from build123d import *

# Parameters (mm, degrees)
EXTRUDE_1_DEPTH = 2


with BuildPart() as part:
    # 草图1 → 凸台-拉伸1 (new body)
    with BuildSketch(Plane.XY):
        with BuildLine():
            Line((-8.45, -5.2), (-8.45, -7))
            Line((-8.45, -7), (12.741644056, -7))
            Line((12.741644056, -7), (13.101478198, -6.889754544))
            Line((13.101478198, -6.889754544), (14.486104816, -6.144709151))
            Line((14.486104816, -6.144709151), (15.312149212, -5.46294768))
            Line((15.312149212, -5.46294768), (14.987866566, -4.436878246))
            Line((14.987866566, -4.436878246), (16.015719748, -4.755461916))
            ThreePointArc((16.015719748, -4.755461916), (17.441105489, -2.542698595), (17.984281104, 0.032763748))
            Line((17.984281104, 0.032763748), (17.029669504, 0.531416269))
            Line((17.029669504, 0.531416269), (17.981499226, 1.035358552))
            ThreePointArc((17.981499226, 1.035358552), (17.266800727, 3.051396039), (15.995852657, 4.771829734))
            Line((15.995852657, 4.771829734), (14.969602225, 4.448120344))
            Line((14.969602225, 4.448120344), (15.288760048, 5.475795391))
            Line((15.288760048, 5.475795391), (14.459323359, 6.1534255))
            Line((14.459323359, 6.1534255), (13.070995905, 6.891551848))
            Line((13.070995905, 6.891551848), (12.710615967, 7))
            Line((12.710615967, 7), (-8.45, 7))
            Line((-8.45, 7), (-8.45, 5.2))
            ThreePointArc((-8.45, 5.2), (-8.308578644, 4.858578644), (-8.65, 5))
            Line((-8.65, 5), (-10.35, 5))
            ThreePointArc((-10.35, 5), (-10.691421356, 4.858578644), (-10.55, 5.2))
            Line((-10.55, 5.2), (-10.55, 7))
            Line((-10.55, 7), (-13, 7))
            Line((-13, 7), (-13, -7))
            Line((-13, -7), (-10.55, -7))
            Line((-10.55, -7), (-10.55, -5.2))
            ThreePointArc((-10.55, -5.2), (-10.691421356, -4.858578644), (-10.35, -5))
            Line((-10.35, -5), (-8.65, -5))
            ThreePointArc((-8.65, -5), (-8.308578644, -4.858578644), (-8.45, -5.2))
        make_face()
        with BuildLine():
            Line((8.461894687, 0.50608965), (4.430504753, 0.50608965))
            Line((4.430504753, 0.50608965), (4.430504753, -0.50608965))
            Line((4.430504753, -0.50608965), (8.461894687, -0.50608965))
            ThreePointArc((8.461894687, -0.50608965), (10.5, -2.1), (12.538105313, -0.50608965))
            Line((12.538105313, -0.50608965), (15.313201547, -0.50608965))
            Line((15.313201547, -0.50608965), (15.313201547, 0.50608965))
            Line((15.313201547, 0.50608965), (12.538105313, 0.50608965))
            ThreePointArc((12.538105313, 0.50608965), (10.5, 2.1), (8.461894687, 0.50608965))
        make_face(mode=Mode.SUBTRACT)
    extrude(amount=EXTRUDE_1_DEPTH)


solid = part.part
The listing builds one solid part. Answer for the finished solid, in the listing's coordinates (mm). A direction names the side the tool comes from. Round coordinates to 2 decimals unless told otherwise and drop trailing zeros. Order: outer loops, then holes, each group sorted by start corner. A loop starts at its lowest first (then second) coordinate and runs counter-clockwise, first axis right, second up. Notation, with made-up numbers: (0.25, 49) -> (30.25, 49) arc R25 ccw to (30.25, 82) -> close; hole circle Ø7 at (25.5, -29). An arc over 180 degrees is marked (long way). Write each question's results on one line, items separated by ' | '. Start each with the question number.
Q1. Which of the six approach directions +Z, -Z, +X, -X, +Y, -Y give full straight-line access (tool end or side, diameter ignored) to faces 4 (the flat face through (-12, 7, 1)), 5 (the cylindrical face through (10.5, 2.1, 1)), 6 (the flat face through (-10, -5, 1))?
Q2. Find section C-C (y = 3.75). Determine the outline of the cut face in (x, z).
Q3. Find section A-A (x = 5.5). Determine the outline of the cut face in (y, z), then the cut area to 3 significant figures.
Q4. The mould has two halves that part along Y. Classify faces 1 (the flat face through (15.313, 0, 1)), 2 (the flat face through (-12, -7, 1)), 3 (the flat face through (13.77, 6.52, 0.99)): pulls with the +Y half, pulls with the -Y half, needs draft (parallel to the pull), parting line crosses it, or undercut.
Q5. Find section B-B (y = -1.5). Determine the outline of the cut face in (x, z).
Q6. Each of these flat-tipped pins is pushed along its axis until it touches: pin 1 (1 mm diameter, centred on y = 5, z = 1.5, fed in from +X); pin 2 (0.5 mm diameter, centred on x = -9.5, z = 1.5, fed in from -Y); pin 3 (0.6 mm diameter, centred on x = 14.5, z = 1, fed in from -Y). Where does it stop, or does it pass through?
Q7. Straight lines are drawn through the part: probe 1 along X at (y, z) = (0, 0.45); probe 2 along Y at (x, z) = (8, 1.2); probe 3 along Y at (x, z) = (-9, 1.15). For each, find the intervals that lie inside material, in ascending order. Write a range as from..to.
Worked answers:
1) face 4: +Z, -Z, +X, -X, +Y | face 5: +Z, -Z | face 6: +Z, -Z, -Y
2) outline: (-13, 0) -> (16.84, 0) -> (16.84, 2) -> (-13, 2) -> close
3) outline: (-7, 0) -> (-0.51, 0) -> (-0.51, 2) -> (-7, 2) -> close; (0.51, 0) -> (7, 0) -> (7, 2) -> (0.51, 2) -> close | area: 26.0 mm2
4) face 1: undercut | face 2: pulls with the -Y half | face 3: pulls with the +Y half
5) outline: (-13, 0) -> (9.03, 0) -> (9.03, 2) -> (-13, 2) -> close; (11.97, 0) -> (17.78, 0) -> (17.78, 2) -> (11.97, 2) -> close
6) pin 1: stops at x = 16.25 | pin 2: stops at y = -5 | pin 3: stops at y = -6.3
7) probe 1: x = -13..4.43, 15.31..17.98 | probe 2: y = -7..-0.51, 0.51..7 | probe 3: y = -5..5
